from build123d import *

# Parameters (mm, degrees)
SKETCH1_R           = 17
BOSS_EXTRUDE1_DEPTH = 1000
SKETCH2_R           = 19
BOSS_EXTRUDE2_DEPTH = 20
BOSS_EXTRUDE3_START = -20
SKETCH3_R           = 19
BOSS_EXTRUDE3_DEPTH = 20
SKETCH4_R           = 10
BOSS_EXTRUDE4_DEPTH = 100


with BuildPart() as part:
    # Sketch1 → Boss-Extrude1 (new body)
    with BuildSketch(Plane.XY):
        Circle(SKETCH1_R)
    extrude(amount=BOSS_EXTRUDE1_DEPTH)

    # Sketch2 → Boss-Extrude2 (add)
    with BuildSketch(Plane.XY.offset(1000)):
        Circle(SKETCH2_R)
    extrude(amount=-BOSS_EXTRUDE2_DEPTH)

    # Sketch3 → Boss-Extrude3 (add)
    with BuildSketch(Plane(origin=(0, 0, 0), x_dir=(-1, 0, 0), z_dir=(0, 0, -1)).offset(BOSS_EXTRUDE3_START)):
        with Locations(Location((0, 0, 0), (0, 0, 180))):
            Circle(SKETCH3_R)
    extrude(amount=BOSS_EXTRUDE3_DEPTH)

    # Sketch4 → Boss-Extrude4 (add)
    with BuildSketch(Plane(origin=(0, 0, 0), x_dir=(1, 0, 0), z_dir=(0, 1, 0))):
        with Locations(Location((0, -500, 0), (0, 0, 270))):
            Circle(SKETCH4_R)
        with Locations(Location((0, -300, 0), (0, 0, 270))):
            Circle(SKETCH4_R)
        with Locations(Location((0, -100, 0), (0, 0, 270))):
            Circle(SKETCH4_R)
        with Locations(Location((0, -700, 0), (0, 0, 270))):
            Circle(SKETCH4_R)
        with Locations(Location((0, -900, 0), (0, 0, 270))):
            Circle(SKETCH4_R)
    extrude(amount=-BOSS_EXTRUDE4_DEPTH)


solid = part.part
Check sheet for the modelled part. Datum: model origin and axes. Units: mm. A direction names the side the tool comes from. Round coordinates to 2 decimals unless told otherwise and drop trailing zeros. Write each loop counter-clockwise with the first axis right and the second up, starting at its lowest first coordinate (ties: lowest second). Pieces come first, ordered by that corner, then holes. Notation, with made-up numbers: (65.5, 82) -> (101.5, 82) arc R34 cw to (101.5, 119) -> close; hole circle Ø1 at (20, -12.5). An arc over 180 degrees is marked (long way). Answer as CSV lines item,"result". Start each with the question number.
1) Material ranges on line 1 (Z direction, x = 2.5, y = -23.5); line 2 (Z direction, x = -2, y = -57); line 3 (Y direction, x = 0, z = 370.5), recorded low to high. Write a range as from..to.
2) Section check C-C on z = 100. Enter the section's corners in (x, y).
3) Go/stop test with flat-tipped pins: P1, Ø10, axis at y = -11.5, z = 484.5, coming from the -X side; P2, Ø6, axis at x = 4, z = 774.5, coming from the -Y side; P3, Ø3, axis at x = -5.5, z = 518, coming from the +Y side. Record where each tip stops, or that it passes through.
4) Section check A-A on y = -44. Enter the section's corners in (x, z).
5) Release check for a two-part mould opening along Z. For faces 4 (the flat face through (0, -100, 300)), 5 (the flat face through (0, 0, 1000)), 6 (the cylindrical face through (3, -56.27, 709.54)) record: pulls with the +Z half, pulls with the -Z half, needs draft (parallel to the pull), parting line crosses it, or undercut.
6) Tool access check on faces 1 (the cylindrical face through (0, -56, 290)), 2 (the cylindrical face through (8.767, -16.856, 990.14)), 3 (the cylindrical face through (9.139, 14.334, 493.28)). Record the directions out of +Z, -Z, +X, -X, +Y, -Y that give a thin tool (end or side, any length) a straight path to the whole face; none if there is none.
Found:
1,line 1,"z = 90.32..109.68, 290.32..309.68, 490.32..509.68, 690.32..709.68, 890.32..909.68"
1,line 2,"z = 90.2..109.8, 290.2..309.8, 490.2..509.8, 690.2..709.8, 890.2..909.8"
1,line 3,"y = -17..17"
2,outline,"(-10, -100) -> (10, -100) -> (10, -13.75) arc R17 ccw (long way) to (-10, -13.75) -> close"
3,P1,"stops at x = -15.71"
3,P2,"stops at y = -16.97"
3,P3,"stops at y = 16.52"
4,outline,"circle Ø20 at (0, 100); circle Ø20 at (0, 300); circle Ø20 at (0, 500); circle Ø20 at (0, 700); circle Ø20 at (0, 900)"
5,face 4,"needs draft"
5,face 5,"pulls with the +Z half"
5,face 6,"undercut"
6,face 1,"-Y"
6,face 2,"+Z"
6,face 3,"none"
